For this review, take the finished solid that the model builds, in its own axes (mm). Give positions to 0.01 mm unless a question says otherwise; leave off trailing zeros. Use a Markdown table: item, result. Add a question column.
1) Wall thickness on L1, parallel to Z at x = -0.75, y = 0.85; L2, parallel to X at y = 0.6, z = -13.25; L3, parallel to Z at x = 0, y = 0.9: over which ranges is each line inside the solid? List them lowest first.
2) Mouldability with a two-part tool opening along Z and no side actions: class faces 1 (the face through (-0.82, 0.79, -14.75)), 2 (the face through (1.22, 0.81, -15.17)), 3 (the face through (1.17, 0.81, 83.22)), 4 (the face through (-1, 1.6, 35)) as released by +Z, released by -Z, zero draft, split by the parting line, or undercut.
3) We need section A-A on y = 1.2. Give the number of separate pieces and of enclosed holes in the cut face, then the cut area to 3 significant figures.
4) Clearance check with a flat-ended pin moving along its axis: P1, Ø3, axis at x = 0, z = 71, coming from the -Y side. State where the tip first meets the part, or that it passes through.
Autodesk Inventor part; units mm, degrees
ref_plane "YZ Plane" through (0, 0, 0) normal (1, 0, 0) x (0, 1, 0)
ref_plane "XZ Plane" through (0, 0, 0) normal (0, 1, 0) x (-1, 0, 0)
ref_plane "XY Plane" through (0, 0, 0) normal (0, 0, 1) x (1, 0, 0)
sketch "Szkic1" plane through (0, 0, 0) normal (0, 1, 0) x (-1, 0, 0)
  line L0 (3.5, 84) -> (-2, 84)
  line L1 (-2, 84) -> (-2, -16)
  line L2 (-2, -16) -> (3.5, -16)
  line L3 (3.5, -16) -> (3.5, 84)
  point P0 (0, 0)
  dimension "d0" = 5.5
  dimension "d1" = 100
extrude "Wyciągnięcie proste1" add sketch "Szkic1" along normal blind 1.6
fillet "Zaokrąglenie1" radius 2.75 4 edges at (-3.5, 0.8, -16) (2, 0.8, -16) (-3.5, 0.8, 84) (2, 0.8, 84)
sketch "Szkic2" plane through (0, 1.6, 0) normal (0, 1, 0) x (1, 0, 0)
  arc A0 (-3.5, -81.25) -> (2, -81.25) centre (-0.75, -81.25) ccw
  line L0 (2, -81.25) -> (2, 13.25)
  arc A1 (2, 13.25) -> (-3.5, 13.25) centre (-0.75, 13.25) ccw
  line L1 (-3.5, 13.25) -> (-3.5, -81.25)
  point P0 (0, 0)
hole "Otwór1" at (-0.75, 1.6, 81.25) at (-0.75, 1.6, -13.25) direction (0, -1, 0) diameter 3 end through all
properties part number "belka"
Checked values:
| question | item | result |
|---|---|---|
| 1 | L1 | -16 to -14.75, -11.75 to 79.75, 82.75 to 84 |
| 1 | L2 | -3.5 to -2.25, 0.75 to 2 |
| 1 | L3 | -15.9 to -14.55, -11.95 to 79.95, 82.55 to 83.9 |
| 2 | face 1 | undercut |
| 2 | face 2 | released by -Z |
| 2 | face 3 | released by +Z |
| 2 | face 4 | zero draft |
| 3 | separate pieces | 1 |
| 3 | enclosed holes | 2 |
| 3 | area | 529 mm² |
| 4 | P1 | y = 0 |
